```python
from build123d import *

# Parameters (mm, degrees)
SKIZZE1_R                       = 11
AUFSATZ_LINEAR_AUSTRAGEN1_DEPTH = 100


with BuildPart() as part:
    # Skizze1 → Aufsatz-Linear austragen1 (new, symmetric)
    with BuildSketch(Plane(origin=(0, 0, 0), x_dir=(0, 0, -1), z_dir=(1, 0, 0))):
        Polygon((-115, 0), (115, 0), (115, -30), (95, -50), (-95, -50), (-115, -30), align=None)
        with Locations((0, -25)):
            Circle(SKIZZE1_R, mode=Mode.SUBTRACT)
        with Locations((-80, -25)):
            Circle(SKIZZE1_R, mode=Mode.SUBTRACT)
        with Locations(Location((80, -25, 0), (0, 0, 180))):
            Circle(SKIZZE1_R, mode=Mode.SUBTRACT)
    extrude(amount=AUFSATZ_LINEAR_AUSTRAGEN1_DEPTH, both=True)


solid = part.part
```
Part model, mm, in its own coordinate system. Round coordinates to 2 decimals unless told otherwise and drop trailing zeros. Loops run counter-clockwise (first coordinate to the right, second up) from the corner with the lowest first, then second, coordinate; pieces in that order, holes last.
Item 1: Cut at B-B, the plane x = 68. Give the cut face in (y, z), then the cut area to 3 significant figures.
Item 2: Cut at D-D, the plane z = 79. Give the cut face in (x, y).
Item 3: Drill centre lines: line 1 (Z direction, x = 39, y = -31); line 2 (Y direction, x = -35, z = 80); line 3 (Z direction, x = -53.5, y = -32.5). Where is each one in solid material? Low to high.
Item 4: Cut at C-C, the plane z = 0. Give the cut face in (x, y).
Item 5: Drop a flat-ended pin along its axis: P1, Ø3, axis at x = -16, y = -38.5, coming from the +Z side. Give the stop position or say it passes through.
Item 6: Mould opens along Y. For faces 1 (the face through (-1.4, -35.74, 2.38)), 2 (the face through (1, -50, -1)), 3 (the face through (1, 0, 2)), 4 (the face through (1, -15, -115)) say: +Y half, -Y half, draft (parallel to the pull), parting line (faces both ways), or undercut.
Item 7: Cut at A-A, the plane y = -25. Give the cut face in (x, z).
A:
1. outline: (-50, -95) - (-30, -115) - (0, -115) - (0, 115) - (-30, 115) - (-50, 95) - close; hole circle Ø22 at (-25, -80); hole circle Ø22 at (-25, 0); hole circle Ø22 at (-25, 80)
1. area: 9,960 mm2
2. outline: (-100, -50) - (100, -50) - (100, -35.95) - (-100, -35.95) - close; (-100, -14.05) - (100, -14.05) - (100, 0) - (-100, 0) - close
3. line 1: z = -114 to -89.22, -70.78 to -9.22, 9.22 to 70.78, 89.22 to 114
3. line 2: y = -50 to -36, -14 to 0
3. line 3: z = -112.5 to -88.05, -71.95 to -8.05, 8.05 to 71.95, 88.05 to 112.5
4. outline: (-100, -50) - (100, -50) - (100, -36) - (-100, -36) - close; (-100, -14) - (100, -14) - (100, 0) - (-100, 0) - close
5. P1: stops at z = 108
6. face 1: undercut
6. face 2: -Y half
6. face 3: +Y half
6. face 4: draft
7. outline: (-100, -115) - (100, -115) - (100, -91) - (-100, -91) - close; (-100, -69) - (100, -69) - (100, -11) - (-100, -11) - close; (-100, 11) - (100, 11) - (100, 69) - (-100, 69) - close; (-100, 91) - (100, 91) - (100, 115) - (-100, 115) - close
